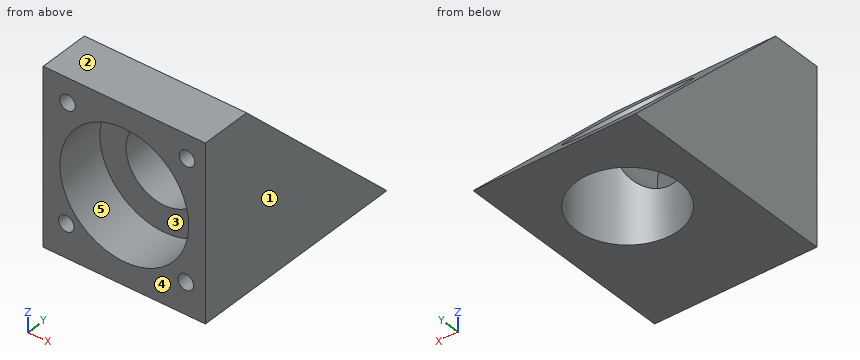
```python
from build123d import *

# Parameters (mm, degrees)
BOSS_EXTRUDE1_DEPTH = 26
SKETCH2_R           = 8.25
CUT_EXTRUDE1_DEPTH  = 29
SKETCH3_R           = 6.15
CUT_EXTRUDE2_DEPTH  = 37.22
SKETCH4_R           = 10.325
SKETCH4_R_2         = 1.25
CUT_EXTRUDE3_DEPTH  = 8


with BuildPart() as part:
    # Sketch1 → Boss-Extrude1 (new body)
    with BuildSketch(Plane(origin=(0, 0, 0), x_dir=(0, 0, -1), z_dir=(1, 0, 0))):
        Polygon((0, 0), (28, 0), (28, 36.22), (0, 8.22), align=None)
    extrude(amount=BOSS_EXTRUDE1_DEPTH)

    # Sketch2 → Cut-Extrude1 (cut, through all)
    with BuildSketch(Plane(origin=(0, 0, -28), x_dir=(-1, 0, 0), z_dir=(0, 0, -1))):
        with Locations((-13, 21.58)):
            Circle(SKETCH2_R)
    extrude(amount=-CUT_EXTRUDE1_DEPTH, mode=Mode.SUBTRACT)

    # Sketch3 → Cut-Extrude2 (cut, through all)
    with BuildSketch(Plane.XZ):
        with Locations((13, -14)):
            Circle(SKETCH3_R)
    extrude(amount=-CUT_EXTRUDE2_DEPTH, mode=Mode.SUBTRACT)

    # Sketch4 → Cut-Extrude3 (cut)
    with BuildSketch(Plane.XZ):
        with Locations((13, -14)):
            Circle(SKETCH4_R)
        with Locations((3.9, -3.85)):
            Circle(SKETCH4_R_2)
        with Locations((23.05, -3.75)):
            Circle(SKETCH4_R_2)
        with Locations((22.85, -22.95)):
            Circle(SKETCH4_R_2)
        with Locations((3.7, -22.65)):
            Circle(SKETCH4_R_2)
    extrude(amount=-CUT_EXTRUDE3_DEPTH, mode=Mode.SUBTRACT)


solid = part.part
```
Can you work these out from the model? Positions are in its coordinate system, mm. Face numbers are marked on the shaded views. A direction names the side the tool comes from. Give positions to 0.01 mm unless a question says otherwise; leave off trailing zeros. Loops run counter-clockwise (first coordinate to the right, second up) from the corner with the lowest first, then second, coordinate; pieces in that order, holes last. Notation, with made-up numbers: M 47,16.5 L 79,16.5 A18 ccw 79,47.5 Z; hole C -3.5,-25 d7. An arc over 180 degrees is marked long. Use one line per item in the form item = value. Start each with the question number.
(1) Thinking about a two-plate mould opening in X: for the marked faces 1, 2 and 3, which applies, released by +X, released by -X, zero draft, split by the parting line, or undercut?
(2) I want a section at B-B, the plane x = 9.75. Write out the boundary of the cut face in (y, z).
(3) On a 3-axis mill with a long thin cutter (end or side, diameter ignored), from which of +Z, -Z, +X, -X, +Y, -Y can I reach the whole of each face in a straight line? I mean the marked faces 4 and 5. Say none if no direction works.
(4) I want a section at C-C, the plane z = -17.25. Write out the boundary of the cut face in (x, y), and give its area (3 significant figures).
(5) I want a section at A-A, the plane y = 26. Write out the boundary of the cut face in (x, z).
(6) Please list where these lines run through material, in increasing order: line 1 (X direction, y = 11.75, z = -14); line 2 (Z direction, x = 3.9, y = 4.25); line 3 (X direction, y = 20, z = -25.75).
(7) I'm going to push flat-ended pins straight in: P1, Ø3, axis at x = 22.85, z = -22.95, coming from the +Y side; P2, Ø3, axis at x = 22, z = -18.5, coming from the +Y side; P3, Ø8, axis at x = 14, y = 23, coming from the +Z side; P4, Ø1.2, axis at x = 3.5, z = -22.5, coming from the -Y side. Where does each tip first touch, or does it pass through?
(8) I want a section at D-D, the plane x = 3.9. Write out the boundary of the cut face in (y, z).
Worked out:
q1.face_1 = released by +X
q1.face_2 = zero draft
q1.face_3 = undercut
q2.outline = M 0,-28 L 14,-28 L 14,-19.22 L 8,-19.22 L 8,-23.8 L 0,-23.8 Z; M 0,-4.2 L 8,-4.2 L 8,-8.78 L 14,-8.78 L 14,-5.78 L 8.22,0 L 0,0 Z; M 29.16,-28 L 36.22,-28 L 29.16,-20.94 Z
q3.face_4 = +Z, -Z, +X, -X, -Y
q3.face_5 = -Y
q4.outline = M 0,0 L 3.2,0 L 3.2,8 L 7.78,8 L 7.78,15.19 A8.25 cw 5.72,25.47 L 0,25.47 Z; M 18.22,8 L 22.8,8 L 22.8,0 L 26,0 L 26,25.47 L 20.28,25.47 A8.25 cw 18.22,15.19 Z
q4.area = 275 mm²
q5.outline = M 0,-28 L 6.03,-28 L 6.03,-17.78 L 0,-17.78 Z; M 19.97,-28 L 26,-28 L 26,-17.78 L 19.97,-17.78 Z
q6.line_1 = 0 to 6.85, 19.15 to 26
q6.line_2 = -28 to -23.88, -21.42 to -18.88, -9.12 to -5.1, -2.6 to 0
q6.line_3 = 0 to 4.9, 21.1 to 26
q7.P1 = 32.67
q7.P2 = 28.22
q7.P3 = through
q7.P4 = 8
q8.outline = M 0,-28 L 36.22,-28 L 8.22,0 L 0,0 L 0,-2.6 L 8,-2.6 L 8,-5.1 L 0,-5.1 L 0,-9.12 L 8,-9.12 L 8,-18.88 L 0,-18.88 L 0,-21.42 L 8,-21.42 L 8,-23.88 L 0,-23.88 Z
